Can you work these out from the model? Positions are in its coordinate system, mm. Face numbers are marked on the shaded views. Coordinates: 2 decimals unless noted, no trailing zeros. Order: outer loops, then holes, each group sorted by start corner. A loop starts at its lowest first (then second) coordinate and runs counter-clockwise, first axis right, second up.
```python
from build123d import *

# Parameters (mm, degrees)
SKETCH1_R           = 1.5113
BOSS_EXTRUDE1_DEPTH = 0.7874
SKETCH2_R           = 1.5875
BOSS_EXTRUDE2_DEPTH = 6.5024
SKETCH3_R           = 1.11850285
CUT_EXTRUDE1_DEPTH  = 2.54


with BuildPart() as part:
    # Sketch1 → Boss-Extrude1 (new body)
    with BuildSketch(Plane(origin=(0, 0, 0), x_dir=(1, 0, 0), z_dir=(0, 1, 0))):
        with BuildLine():
            Line((-6.468656663, -1.40130078), (-9.301119213, -1.016))
            Line((-9.301119213, -1.016), (-14.224, -1.016))
            Line((-14.224, -1.016), (-14.224, 0))
            Line((-14.224, 0), (-14.224, 1.016))
            Line((-14.224, 1.016), (-9.301119213, 1.016))
            Line((-9.301119213, 1.016), (-6.468656663, 1.40130078))
            ThreePointArc((-6.468656663, 1.40130078), (-3.615678691, 1.908544578), (-0.813473119, 2.646395179))
            ThreePointArc((-0.813473119, 2.646395179), (2.7686, 0), (-0.813473119, -2.646395179))
            ThreePointArc((-0.813473119, -2.646395179), (-3.615678691, -1.908544578), (-6.468656663, -1.40130078))
        make_face()
        with Locations(Location((0, 0, 0), (0, 0, 270))):
            Circle(SKETCH1_R, mode=Mode.SUBTRACT)
    extrude(amount=BOSS_EXTRUDE1_DEPTH)

    # Sketch2 → Boss-Extrude2 (add)
    with BuildSketch(Plane.ZY.offset(14.224)):
        with Locations((0, 1.219795167)):
            Circle(SKETCH2_R)
    extrude(amount=-BOSS_EXTRUDE2_DEPTH)

    # Sketch3 → Cut-Extrude1 (cut)
    with BuildSketch(Plane.ZY.offset(14.224)):
        with Locations((0, 1.219795167)):
            Circle(SKETCH3_R)
    extrude(amount=-CUT_EXTRUDE1_DEPTH, mode=Mode.SUBTRACT)


solid = part.part
```
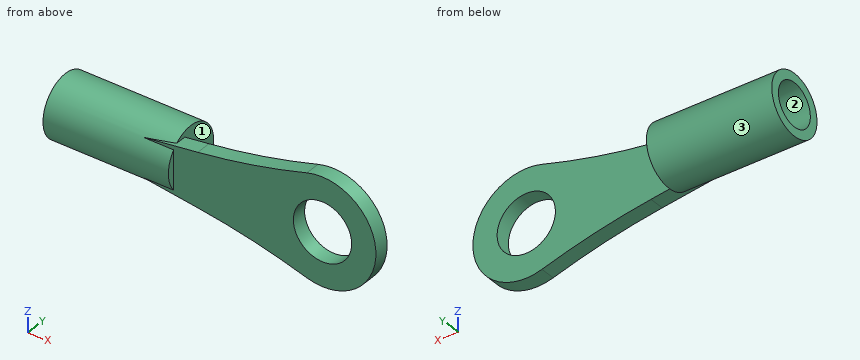
1. Imagine slicing it at B-B on x = 0.5. Please give me the cut outline in (y, z).
Completed:
outline: (0, -2.72) - (0.79, -2.72) - (0.79, -1.43) - (0, -1.43) - close; (0, 1.43) - (0.79, 1.43) - (0.79, 2.72) - (0, 2.72) - close
2. I'm going to push flat-ended pins straight in: pin 1 (1.5 mm diameter, centred on y = 0, z = 0.5, fed in from +X); pin 2 (1.7 mm diameter, centred on x = -2.5, z = 0, fed in from -Y); pin 3 (1.5 mm diameter, centred on x = -1, y = 0.5, fed in from -Z); pin 4 (1 mm diameter, centred on x = -9.5, y = 0.5, fed in from -Z). Where does each tip first touch, or does it pass through?
Completed:
pin 1: stops at x = 2.77
pin 2: stops at y = 0
pin 3: stops at z = -2.76
pin 4: stops at z = -1.57
3. Imagine slicing it at A-A on z = 0. Please give me the cut outline in (x, y), then the cut area to 3 significant figures.
Completed:
outline: (-14.22, -0.37) - (-7.72, -0.37) - (-7.72, 0) - (-1.51, 0) - (-1.51, 0.79) - (-7.72, 0.79) - (-7.72, 2.81) - (-14.22, 2.81) - (-14.22, 2.34) - (-11.68, 2.34) - (-11.68, 0.1) - (-14.22, 0.1) - close; (1.51, 0) - (2.77, 0) - (2.77, 0.79) - (1.51, 0.79) - close
area: 20.8 mm2
4. Imagine slicing it at C-C on y = 1.6. Please give me the cut outline in (x, z), then the cut area to 3 significant figures.
Completed:
outline: (-14.22, -1.54) - (-7.72, -1.54) - (-7.72, 1.54) - (-14.22, 1.54) - (-14.22, 1.05) - (-11.68, 1.05) - (-11.68, -1.05) - (-14.22, -1.05) - close
area: 14.7 mm2
5. Thinking about a two-plate mould opening in Z: for the marked faces 1, 2 and 3, which applies, pulls with the +Z half, pulls with the -Z half, needs draft (parallel to the pull), parting line crosses it, or undercut?
Completed:
face 1: needs draft
face 2: undercut
face 3: parting line crosses it
6. Please list where these lines run through material, in increasing order: probe 1 along X at (y, z) = (0.25, 0); probe 2 along X at (y, z) = (-0.2, -0.1); probe 3 along Y at (x, z) = (0.25, -1.9).
Completed:
probe 1: x = -11.68 to -1.51, 1.51 to 2.77
probe 2: x = -14.22 to -7.72
probe 3: y = 0 to 0.79
7. Imagine slicing it at D-D on y = 0.4. Please give me the cut outline in (x, z), then the cut area to 3 significant figures.
Completed:
outline: (-14.22, -1.36) - (-7.72, -1.36) - (-7.72, -1.23) - (-6.47, -1.4) arc R35.56 cw to (-0.81, -2.65) arc R2.77 ccw (long way) to (-0.81, 2.65) arc R35.56 cw to (-6.47, 1.4) - (-7.72, 1.23) - (-7.72, 1.36) - (-14.22, 1.36) - (-14.22, 0.76) - (-11.68, 0.76) - (-11.68, -0.76) - (-14.22, -0.76) - close; hole circle Ø3.02 at (0, 0)
area: 48.4 mm2
